from build123d import *

# Parameters (mm, degrees)
CROQUIS2_R = 3


with BuildPart() as part:
    # Barrer1: sweep along a path in Croquis1
    with BuildLine(Plane(origin=(0, 0, 0), x_dir=(1, 0, 0), z_dir=(0, 1, 0))) as barrer1_path:
        Line((0, 0), (0, 7))
        ThreePointArc((0, 7), (1.146798787, 10.839275396), (4.211438733, 13.420586115))
        Line((4.211438733, 13.420586115), (75.016341047, 44.172265879))
        ThreePointArc((75.016341047, 44.172265879), (84.484679137, 43.361716018), (89, 35))
        Line((89, 35), (89, 22))
    # Croquis2 → Barrer1 (sweep)
    with BuildSketch(Plane.XY):
        Circle(CROQUIS2_R)
    barrer1 = sweep(path=barrer1_path.line)

    # Simetría1: Barrer1 across plane
    add(barrer1.mirror(Plane.XY))


solid = part.part
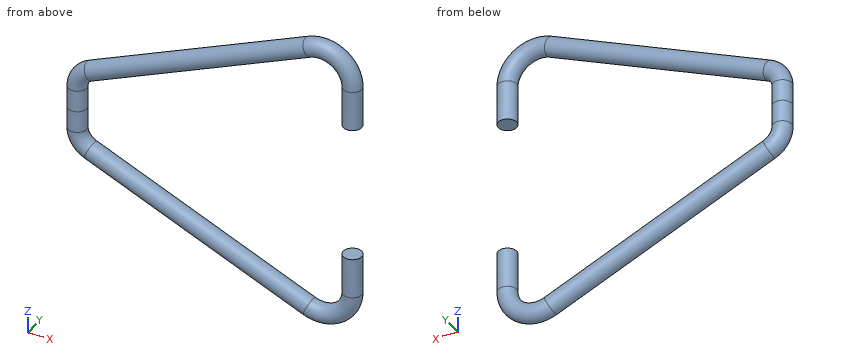
Source: CAD feature listing. Evaluate the final solid. Frame: model axes, mm. Give positions to 0.01 mm unless a question says otherwise; leave off trailing zeros. Write each loop counter-clockwise with the first axis right and the second up, starting at its lowest first coordinate (ties: lowest second). Pieces come first, ordered by that corner, then holes. Notation, with made-up numbers: (45, 31) -> (86, 31) arc R27 ccw to (86, 59) -> close; hole circle Ø8 at (-19.75, -31). An arc over 180 degrees is marked (long way). Return JSON: item names as keys, results as strings. Group by question number.
1. Section B-B, the plane y = 0. Output: boundary loops of the cut face in (x, z), then the cut area to 3 significant figures.
2. Section A-A, the plane z = -4. Output: boundary loops of the cut face in (x, y), then the cut area to 3 significant figures.
3. Pin query (flat end, axial travel): pin 1 Ø2 at (x, y) = (19, 1) entering from -Z; pin 2 Ø3 at (x, y) = (90, 0) entering from -Z; pin 3 Ø1 at (x, y) = (39.5, 2) entering from +Z. Return the tip coordinate at first contact, or that it passes through.
4. Material intervals for line 1 (Z direction, x = 55.5, y = -2.5); line 2 (Z direction, x = 32, y = 2.5); line 3 (X direction, y = 2, z = 38), sorted ascending. Write a range as from..to.
Determined:
{
 "1": {"outline": "(-3, -7) arc R10 ccw to (3.02, -16.17) -> (73.82, -46.92) arc R13 ccw to (92, -35) -> (92, -22) -> (86, -22) -> (86, -35) arc R7 cw to (76.21, -41.42) -> (5.41, -10.67) arc R4 cw to (3, -7) -> (3, 7) arc R4 cw to (5.41, 10.67) -> (76.21, 41.42) arc R7 cw to (86, 35) -> (86, 22) -> (92, 22) -> (92, 35) arc R13 ccw to (73.82, 46.92) -> (3.02, 16.17) arc R10 ccw to (-3, 7) -> close", "area": "1,500 mm2"},
 "2": {"outline": "circle Ø6 at (0, 0)", "area": "28.3 mm2"},
 "3": {"pin 1": "stops at z = -23.45", "pin 2": "stops at z = -43.87", "pin 3": "stops at z = 31.65"},
 "4": {"line 1": "z = -37.5..-33.89, 33.89..37.5", "line 2": "z = -27.3..-23.68, 23.68..27.3", "line 3": "x = 55.19..66.42, 86.16..90.86"}
}
